Study the drawing (mm; zero at the part's minimum x, y, z) and answer. Give positions to 0.01 mm unless a question says otherwise; leave off trailing zeros. Order: outer loops, then holes, each group sorted by start corner. A loop starts at its lowest first (then second) coordinate and runs counter-clockwise, first axis right, second up.
Item 1: The mould has two halves that part along Z. Classify the marked faces 1, 2 and 3: +Z half, -Z half, draft (parallel to the pull), parting line (faces both ways), or undercut.
Item 2: A cutting plane is placed at A-A (x = 5.5). Write down the section's boundary in (y, z) (1 decimal), plus the area to 3 significant figures.
Item 3: Find the intervals of material crossed by line 1 along X through (y, z) = (8, 15.75); line 2 along Y through (x, z) = (12, 13.25) (1 decimal); line 3 along Y through (x, z) = (12.5, 12.7) (1 decimal), in increasing order.
Item 4: A cutting plane is placed at B-B (z = 9). State how many separate pieces and enclosed holes the cut face has, plus the area to 3 significant figures.
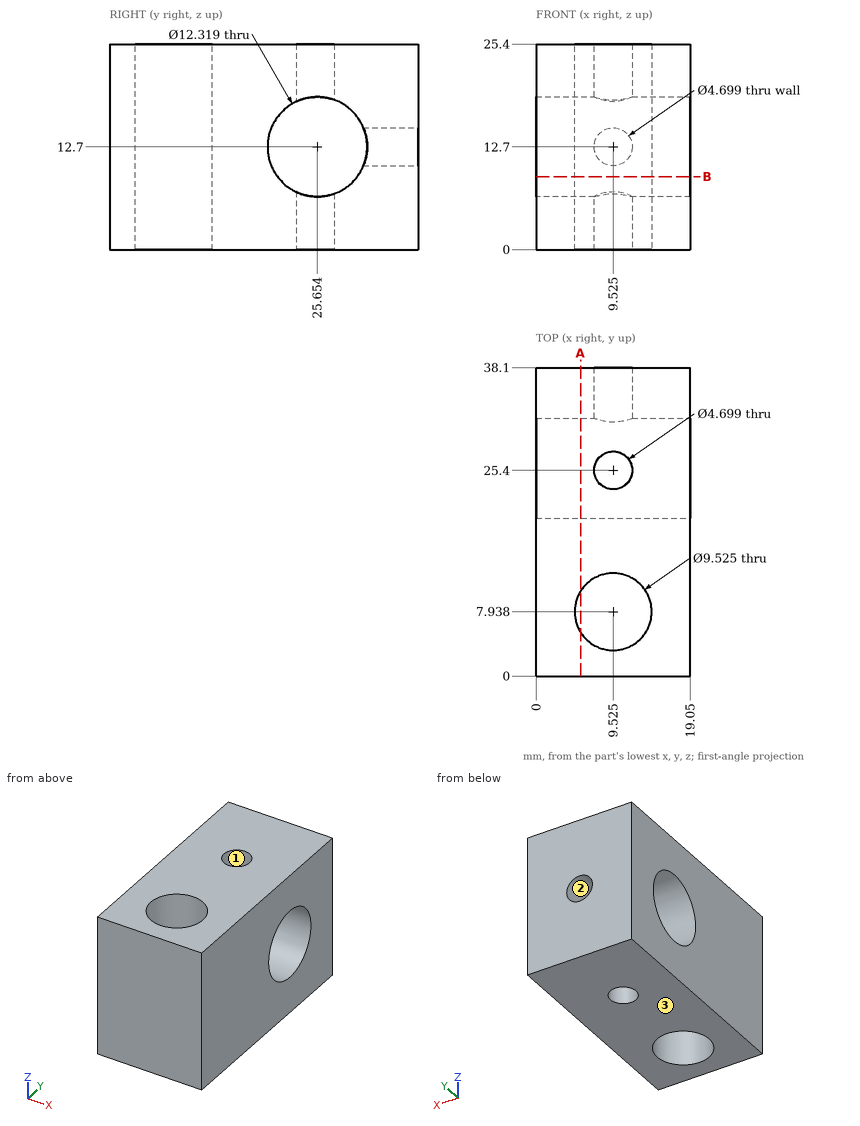
Response values:
1. face 1: draft
1. face 2: undercut
1. face 3: -Z half
2. outline: (0, 0) - (5.4, 0) - (5.4, 25.4) - (0, 25.4) - close; (10.5, 0) - (38.1, 0) - (38.1, 25.4) - (10.5, 25.4) - close; hole circle Ø12.3 at (25.7, 12.7)
2. area: 719 mm2
3. line 1: x = 0 to 4.76, 14.29 to 19.05
3. line 2: y = 0 to 3.9, 12 to 19.5, 31.8 to 38.1
3. line 3: y = 0 to 4.2, 11.7 to 19.5, 31.8 to 38.1
4. separate pieces: 2
4. enclosed holes: 1
4. area: 467 mm2
